```python
from build123d import *

# Parameters (mm, degrees)
SKETCH1_W                = 55
SKETCH1_H                = 20
BOSS_EXTRUDE1_DEPTH      = 7
SKETCH4_R                = 2.5
CUT_EXTRUDE3_DEPTH       = 1
SKETCH5_R                = 1.5
CUT_EXTRUDE4_DEPTH       = 41.197383539
SKETCH6_W                = 7
SKETCH6_H                = 20
BOSS_EXTRUDE2_DEPTH      = 18
SKETCH7_R                = 2.15
CUT_EXTRUDE5_DEPTH       = 7
SKETCH11_R               = 2.15
CUT_EXTRUDE6_DEPTH       = 7
SKETCH12_W               = 55
SKETCH12_H               = 25
BOSS_EXTRUDE3_DEPTH      = 2
SKETCH13_W               = 55
SKETCH13_H               = 25
BOSS_EXTRUDE4_DEPTH      = 2
SKETCH15_W               = 24
SKETCH15_H               = 25
BOSS_EXTRUDE5_DEPTH      = 10
SKETCH29_W               = 65
SKETCH29_H               = 24
CUT_EXTRUDE20_DEPTH      = 5
CUT_EXTRUDE21_DEPTH      = 45.585083194
CUT_EXTRUDE21_DEPTH_BACK = 45.585083194
SKETCH30_R               = 2
SKETCH31_R               = 3.5
CUT_EXTRUDE22_DEPTH      = 45.585083194
SKETCH32_W               = 24
SKETCH32_H               = 20
CUT_EXTRUDE23_DEPTH      = 7
SKETCH33_R               = 2.15
CUT_EXTRUDE24_DEPTH      = 43.811559694
SKETCH35_W               = 7
SKETCH35_H               = 2
CUT_EXTRUDE26_DEPTH      = 17


with BuildPart() as part:
    # Sketch1 → Boss-Extrude1 (new body)
    with BuildSketch(Plane(origin=(0, 0, 0), x_dir=(1, 0, 0), z_dir=(0, 1, 0))):
        with Locations((-6.848648349, 10)):
            Rectangle(SKETCH1_W, SKETCH1_H)
    extrude(amount=BOSS_EXTRUDE1_DEPTH)

    # Sketch4 → Cut-Extrude3 (cut)
    with BuildSketch(Plane(origin=(0, 7, 0), x_dir=(1, 0, 0), z_dir=(0, 1, 0))):
        with Locations(Location((-17.348648349, 10, 0), (0, 0, 270))):
            Circle(SKETCH4_R)
    extrude(amount=-CUT_EXTRUDE3_DEPTH, mode=Mode.SUBTRACT)

    # Sketch5 → Cut-Extrude4 (cut, through all)
    with BuildSketch(Plane(origin=(0, 6, 0), x_dir=(1, 0, 0), z_dir=(0, 1, 0))):
        with Locations(Location((-17.348648349, 10, 0), (0, 0, 270))):
            Circle(SKETCH5_R)
    extrude(amount=-CUT_EXTRUDE4_DEPTH, mode=Mode.SUBTRACT)

    # Sketch6 → Boss-Extrude2 (add)
    with BuildSketch(Plane(origin=(0, 0, 0), x_dir=(-1, 0, 0), z_dir=(0, -1, 0))):
        with Locations((30.848648349, 10)):
            Rectangle(SKETCH6_W, SKETCH6_H)
        with Locations((-17.151351651, 10)):
            Rectangle(SKETCH6_W, SKETCH6_H)
    extrude(amount=BOSS_EXTRUDE2_DEPTH)

    # Sketch7 → Cut-Extrude5 (cut)
    with BuildSketch(Plane(origin=(0, -18, 0), x_dir=(-1, 0, 0), z_dir=(0, -1, 0))):
        with Locations(Location((31.298648349, 15.65, 0), (0, 0, 90))):
            Circle(SKETCH7_R)
        with Locations(Location((31.298648349, 4.35, 0), (0, 0, 90))):
            Circle(SKETCH7_R)
    extrude(amount=-CUT_EXTRUDE5_DEPTH, mode=Mode.SUBTRACT)

    # Sketch11 → Cut-Extrude6 (cut)
    with BuildSketch(Plane(origin=(0, -18, 0), x_dir=(-1, 0, 0), z_dir=(0, -1, 0))):
        with Locations(Location((-17.101351651, 15.65, 0), (0, 0, 90))):
            Circle(SKETCH11_R)
        with Locations(Location((-17.101351651, 4.35, 0), (0, 0, 90))):
            Circle(SKETCH11_R)
    extrude(amount=-CUT_EXTRUDE6_DEPTH, mode=Mode.SUBTRACT)

    # Sketch12 → Boss-Extrude3 (add)
    with BuildSketch(Plane.XY):
        with Locations((-6.848648349, -5.5)):
            Rectangle(SKETCH12_W, SKETCH12_H)
    extrude(amount=BOSS_EXTRUDE3_DEPTH)

    # Sketch13 → Boss-Extrude4 (add)
    with BuildSketch(Plane(origin=(0, 0, -20), x_dir=(-1, 0, 0), z_dir=(0, 0, -1))):
        with Locations((6.848648349, -5.5)):
            Rectangle(SKETCH13_W, SKETCH13_H)
    extrude(amount=BOSS_EXTRUDE4_DEPTH)

    # Sketch15 → Boss-Extrude5 (add)
    with BuildSketch(Plane(origin=(20.651351651, 0, 0), x_dir=(0, 0, -1), z_dir=(1, 0, 0))):
        with Locations((10, -5.5)):
            Rectangle(SKETCH15_W, SKETCH15_H)
    extrude(amount=BOSS_EXTRUDE5_DEPTH)

    # Sketch29 → Cut-Extrude20 (cut)
    with BuildSketch(Plane(origin=(0, 7, 0), x_dir=(1, 0, 0), z_dir=(0, 1, 0))):
        with Locations((-1.848648349, 10)):
            Rectangle(SKETCH29_W, SKETCH29_H)
    extrude(amount=-CUT_EXTRUDE20_DEPTH, mode=Mode.SUBTRACT)

    # Sketch30 → Cut-Extrude21 (cut, two sides: drawn at the far end of the back side and taken through both)
    with BuildSketch(Plane(origin=(0, 0, 0), x_dir=(-1, 0, 0), z_dir=(0, 0, -1)).offset(-CUT_EXTRUDE21_DEPTH_BACK)):
        with Locations((17.348648349, -5)):
            Circle(SKETCH30_R)
    extrude(amount=CUT_EXTRUDE21_DEPTH + CUT_EXTRUDE21_DEPTH_BACK, mode=Mode.SUBTRACT)

    # Sketch31 → Cut-Extrude22 (cut, through all)
    with BuildSketch(Plane.XZ):
        with Locations(Location((-17.348648349, -10, 0), (0, 0, 270))):
            Circle(SKETCH31_R)
    extrude(amount=-CUT_EXTRUDE22_DEPTH, mode=Mode.SUBTRACT)

    # Sketch32 → Cut-Extrude23 (cut)
    with BuildSketch(Plane(origin=(30.651351651, 0, 0), x_dir=(0, 0, -1), z_dir=(1, 0, 0))):
        with Locations((10, -8)):
            Rectangle(SKETCH32_W, SKETCH32_H)
    extrude(amount=-CUT_EXTRUDE23_DEPTH, mode=Mode.SUBTRACT)

    # Sketch33 → Cut-Extrude24 (cut, through all)
    with BuildSketch(Plane.XZ.offset(11)):
        with Locations(Location((17.101351651, -15.65, 0), (0, 0, 270))):
            Circle(SKETCH33_R)
        with Locations(Location((17.101351651, -4.35, 0), (0, 0, 270))):
            Circle(SKETCH33_R)
        with Locations(Location((-31.298648349, -15.65, 0), (0, 0, 270))):
            Circle(SKETCH33_R)
        with Locations(Location((-31.298648349, -4.35, 0), (0, 0, 270))):
            Circle(SKETCH33_R)
    extrude(amount=-CUT_EXTRUDE24_DEPTH, mode=Mode.SUBTRACT)

    # Sketch35 → Cut-Extrude26 (cut)
    with BuildSketch(Plane.XZ.offset(18)):
        with Locations((-30.848648349, -9)):
            Rectangle(SKETCH35_W, SKETCH35_H)
        with Locations((-30.848648349, -11)):
            Rectangle(SKETCH35_W, SKETCH35_H)
    extrude(amount=-CUT_EXTRUDE26_DEPTH, mode=Mode.SUBTRACT)


solid = part.part
```
Read the model definition and answer for the solid it produces. Units are mm, in the model's axes. A direction names the side the tool comes from. Round coordinates to 2 decimals unless told otherwise and drop trailing zeros. Write each loop counter-clockwise with the first axis right and the second up, starting at its lowest first coordinate (ties: lowest second). Pieces come first, ordered by that corner, then holes. Notation, with made-up numbers: (3.5, 32.25) -> (36.5, 32.25) arc R18 cw to (36.5, 67.25) -> close; hole circle Ø11 at (-3, 52.5). An arc over 180 degrees is marked (long way). Answer in a Markdown table with one row per item. Add a question column.
1) Given P1, Ø3, axis at x = -17.35, y = -5, coming from the -Z side; P2, Ø1, axis at x = -15.5, z = -4, coming from the -Y side, each flat-ended and moving along its own axis, determine where each tip first touches the part or whether it passes through.
2) Find section C-C, the plane z = -10. Determine the outline of the cut face in (x, y).
3) Find section A-A, the plane z = -15.65. Determine the outline of the cut face in (x, y).
4) Find section D-D, the plane y = -9.5. Determine the outline of the cut face in (x, z).
5) Determine the mould class of faces 4 (the face through (-7, 0, -10)), 5 (the face through (-19.256, -4.399, -20.986)), 6 (the face through (-19.478, 0.986, -7.223)), 7 (the face through (-6, 2, -10)) for opening direction Y: pulls with the +Y half, pulls with the -Y half, needs draft (parallel to the pull), parting line crosses it, or undercut.
6) Consider line 1 (X direction, y = -10.5, z = -15.65); line 2 (X direction, y = -9.25, z = -15.5); line 3 (X direction, y = -3, z = -19.75). Determine where each line is inside the solid, lowest interval first.
7) Find section B-B, the plane y = -6. Determine the outline of the cut face in (x, z).
8) Which of the six approach directions +Z, -Z, +X, -X, +Y, -Y give full straight-line access (tool end or side, diameter ignored) to faces 1 (the face through (-31, -10, -12)), 2 (the face through (-6, -8, 2)), 3 (the face through (-27.349, -8.9, -7.6))?
Findings below:
| question | item | result |
|---|---|---|
| 1 | P1 | through |
| 1 | P2 | y = 0 |
| 2 | outline | (-34.35, -1) -> (-27.35, -1) -> (-27.35, 0) -> (-20.85, 0) -> (-20.85, 2) -> (-34.35, 2) -> close; (-13.85, 0) -> (13.65, 0) -> (13.65, -18) -> (23.65, -18) -> (23.65, 2) -> (-13.85, 2) -> close |
| 3 | outline | (-34.35, -18) -> (-33.45, -18) -> (-33.45, 2) -> (-34.35, 2) -> close; (-29.15, -18) -> (-27.35, -18) -> (-27.35, 0) -> (13.65, 0) -> (13.65, -18) -> (14.95, -18) -> (14.95, 2) -> (-29.15, 2) -> close; (19.25, -18) -> (23.65, -18) -> (23.65, 2) -> (19.25, 2) -> close |
| 4 | outline | (-34.35, -22) -> (23.65, -22) -> (23.65, 2) -> (-34.35, 2) -> (-34.35, -8) -> (-27.35, -8) -> (-27.35, 0) -> (13.65, 0) -> (13.65, -20) -> (-27.35, -20) -> (-27.35, -12) -> (-34.35, -12) -> close; hole circle Ø4.3 at (-31.3, -15.65); hole circle Ø4.3 at (-31.3, -4.35); hole circle Ø4.3 at (17.1, -15.65); hole circle Ø4.3 at (17.1, -4.35) |
| 5 | face 4 | pulls with the -Y half |
| 5 | face 5 | undercut |
| 5 | face 6 | needs draft |
| 5 | face 7 | pulls with the +Y half |
| 6 | line 1 | -34.35 to -33.45, -29.15 to -27.35, 13.65 to 14.95, 19.25 to 23.65 |
| 6 | line 2 | -34.35 to -33.44, -29.15 to -27.35, 13.65 to 14.96, 19.25 to 23.65 |
| 6 | line 3 | -34.35 to -27.35, 13.65 to 23.65 |
| 7 | outline | (-34.35, -22) -> (-19.08, -22) -> (-19.08, -20) -> (-27.35, -20) -> (-27.35, -12) -> (-34.35, -12) -> close; (-34.35, -8) -> (-27.35, -8) -> (-27.35, 0) -> (-19.08, 0) -> (-19.08, 2) -> (-34.35, 2) -> close; (-15.62, -22) -> (23.65, -22) -> (23.65, 2) -> (-15.62, 2) -> (-15.62, 0) -> (13.65, 0) -> (13.65, -20) -> (-15.62, -20) -> close; hole circle Ø4.3 at (-31.3, -15.65); hole circle Ø4.3 at (-31.3, -4.35); hole circle Ø4.3 at (17.1, -15.65); hole circle Ø4.3 at (17.1, -4.35) |
| 8 | face 1 | -X, -Y |
| 8 | face 2 | +Z, +X, -X, +Y, -Y |
| 8 | face 3 | -Y |
